For this review, use the dimensioned drawing (mm, ordinates from the lowest corner) and the shaded views. A direction names the side the tool comes from. Coordinates: 2 decimals unless noted, no trailing zeros. Loops run counter-clockwise (first coordinate to the right, second up) from the corner with the lowest first, then second, coordinate; pieces in that order, holes last. Notation, with made-up numbers: M 11.5,79.5 L 43.5,79.5 A33 ccw 43.5,115.5 Z; hole C -13,11 d10. An arc over 180 degrees is marked long. Use CSV: the item, a comma, the result in double quotes. Start each with the question number.
1. Add section A-A, the plane y = 2.75. Write out the cut boundary in (x, z), then the cut area to 3 significant figures.
2. Tool access review of the marked faces 1 and 2: name each direction out of +Z, -Z, +X, -X, +Y, -Y from which nothing blocks a thin tool from reaching the whole face with its end or side.
3. Add section C-C, the plane x = 0.55. Write out the cut boundary in (y, z).
4. Add section D-D, the plane z = 13.25. Write out the cut boundary in (x, y).
5. For L1, parallel to X at y = 3.15, z = 11 (1 decimal); L2, parallel to Z at x = 4.45, y = 3, list the stretches that pass through material, from the lowest coordinate up.
6. Add section B-B, the plane z = 7. Write out the cut boundary in (x, y).
7. Draft analysis for pull direction Y (two halves, no side actions). For the marked faces 3, 4 and 5, state which applies: +Y half, -Y half, draft (parallel to the pull), parting line (faces both ways), or undercut.
8. Clearance check with flat-ended pins moving along their axes: P1, Ø1.5, axis at y = 3.5, z = 2, coming from the -X side; P2, Ø3, axis at y = 3.5, z = 6, coming from the +X side; P3, Ø1.5, axis at x = 3.5, z = 10, coming from the +Y side. State where each tip first meets the part, or that it passes through.
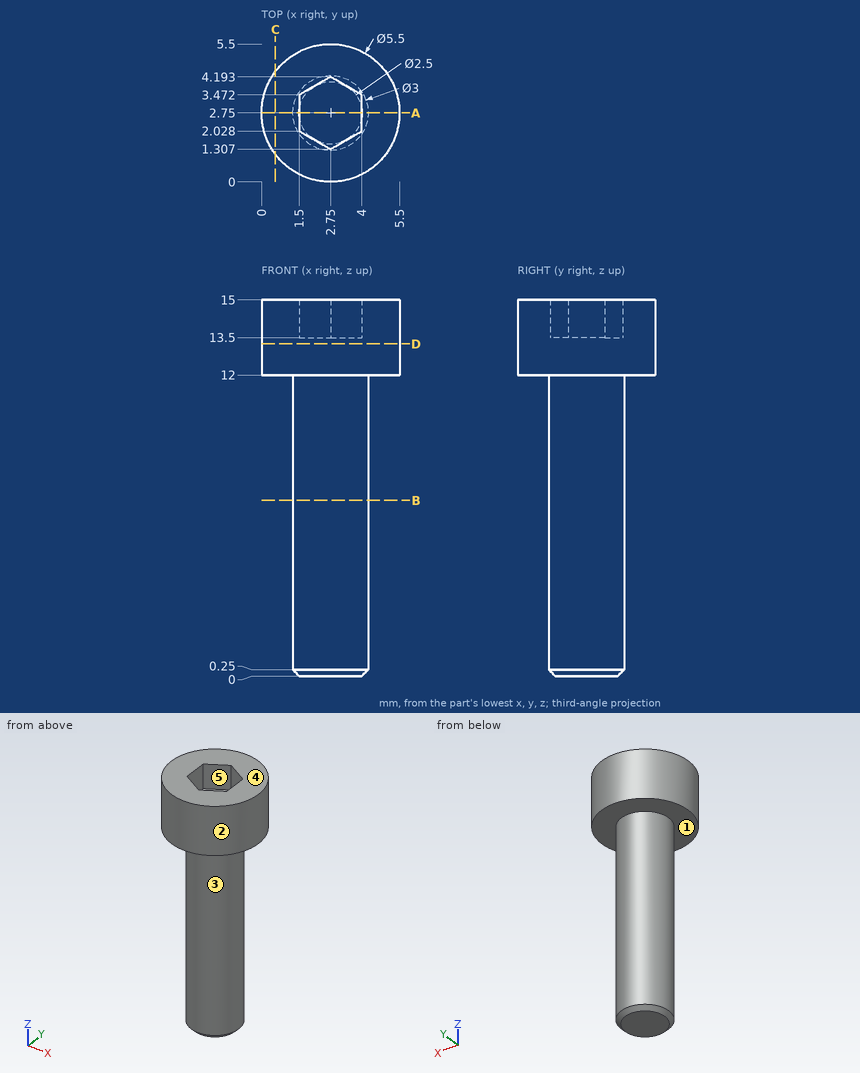
Computed:
1,outline,"M 0,12 L 1.25,12 L 1.25,0.25 L 1.5,0 L 4,0 L 4.25,0.25 L 4.25,12 L 5.5,12 L 5.5,15 L 4,15 L 4,13.5 L 1.5,13.5 L 1.5,15 L 0,15 Z"
1,area,"48.7 mm^2"
2,face 1,"-Z"
2,face 2,"+Z, -Z"
3,outline,"M 1.1,12 L 4.4,12 L 4.4,15 L 1.1,15 Z"
4,outline,"C 2.75,2.75 d5.5"
5,L1,"x = 1.3 to 4.2"
5,L2,"z = 12 to 15"
6,outline,"C 2.75,2.75 d3"
7,face 3,"parting line"
7,face 4,"draft"
7,face 5,"undercut"
8,P1,"stops at x = 1.25"
8,P2,"stops at x = 4.25"
8,P3,"stops at y = 4.25"
